from build123d import *
from build123d.topology import SkipClean

# Parameters (mm, degrees)
SKETCH1_R           = 50.8
SKETCH1_R_2         = 44.45
BOSS_EXTRUDE1_DEPTH = 6.35
BOSS_EXTRUDE2_DEPTH = 95.25


with BuildPart() as part:
    # Sketch1 → Boss-Extrude1 (new body)
    with BuildSketch(Plane(origin=(0, 0, 0), x_dir=(1, 0, 0), z_dir=(0, 1, 0))):
        with Locations(Location((0, 0, 0), (0, 0, 270))):
            Circle(SKETCH1_R)
        with Locations(Location((0, 0, 0), (0, 0, 270))):
            Circle(SKETCH1_R_2, mode=Mode.SUBTRACT)
    extrude(amount=BOSS_EXTRUDE1_DEPTH)

    # Sketch2 → Boss-Extrude2 (add)
    with SkipClean():  # the faces are left unmerged after this step: merging them gives an invalid solid
        with BuildSketch(Plane(origin=(0, 6.35, 0), x_dir=(1, 0, 0), z_dir=(0, 1, 0))):
            with BuildLine():
                ThreePointArc((0, 50.8), (-3.863527606, 50.652869163), (-7.704675524, 50.212328915))
                Line((-7.704675524, 50.212328915), (-7.704675524, 43.777168422))
                ThreePointArc((-7.704675524, 43.777168422), (-3.866999071, 44.281472629), (0, 44.45))
                Line((0, 44.45), (0, 50.8))
            make_face()
        extrude(amount=BOSS_EXTRUDE2_DEPTH)


solid = part.part
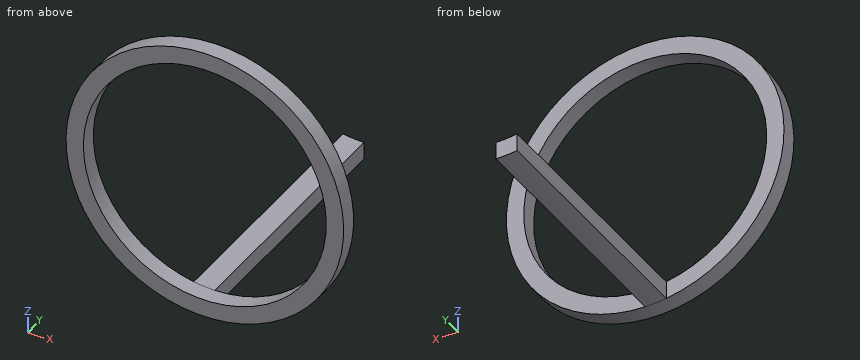
The listing builds one solid part. Answer for the finished solid, in the listing's coordinates (mm). Round coordinates to 2 decimals unless told otherwise and drop trailing zeros. Order: outer loops, then holes, each group sorted by start corner. A loop starts at its lowest first (then second) coordinate and runs counter-clockwise, first axis right, second up. Notation, with made-up numbers: M 70.25,89.25 L 97.25,89.25 A14 ccw 97.25,103.25 Z; hole C 36.25,21 d9. An arc over 180 degrees is marked long. Answer in a Markdown table with one row per item. Add a question column.
1) The part is cut by section A-A on z = 0. Determine the outline of the cut face in (x, y).
2) Consider line 1 along X through (y, z) = (3, 0); line 2 along X through (y, z) = (55.5, -46); line 3 along Y through (x, z) = (-17, 46). Determine where each line is inside the solid, lowest interval first. Write a range as from..to.
3) The part is cut by section B-B on x = 21. Determine the outline of the cut face in (y, z), plus the area to 3 significant figures.
4) Flat-ended cylindrical pins translate along their axes: pin 1 Ø3 at (y, z) = (50, -47) entering from +X; pin 2 Ø2 at (x, y) = (-2.5, 11.5) entering from -Z; pin 3 Ø7 at (y, z) = (75.5, -48) entering from -X. Find the tip coordinate at first contact, or state that the pin passes through.
5) The part is cut by section C-C on y = 67. Determine the outline of the cut face in (x, z), plus the area to 3 significant figures.
Findings below:
| question | item | result |
|---|---|---|
| 1 | outline | M -50.8,0 L -44.45,0 L -44.45,6.35 L -50.8,6.35 Z; M 44.45,0 L 50.8,0 L 50.8,6.35 L 44.45,6.35 Z |
| 2 | line 1 | x = -50.8..-44.45, 44.45..50.8 |
| 2 | line 2 | x = -7.7..0 |
| 2 | line 3 | y = 0..6.35 |
| 3 | outline | M 0,-46.26 L 6.35,-46.26 L 6.35,-39.18 L 0,-39.18 Z; M 0,39.18 L 6.35,39.18 L 6.35,46.26 L 0,46.26 Z |
| 3 | area | 89.9 mm² |
| 4 | pin 1 | stops at x = 0 |
| 4 | pin 2 | stops at z = -50.78 |
| 4 | pin 3 | stops at x = -7.7 |
| 5 | outline | M -7.7,-50.21 A50.8 ccw 0,-50.8 L 0,-44.45 A44.45 cw -7.7,-43.78 Z |
| 5 | area | 49.1 mm² |
